Source: CAD feature listing. Evaluate the final solid. Frame: model axes, mm. A direction names the side the tool comes from. Give positions to 0.01 mm unless a question says otherwise; leave off trailing zeros. Write each loop counter-clockwise with the first axis right and the second up, starting at its lowest first coordinate (ties: lowest second). Pieces come first, ordered by that corner, then holes.
Autodesk Inventor part; units mm, degrees
ref_plane "YZ Plane" through (0, 0, 0) normal (1, 0, 0) x (0, 1, 0)
ref_plane "XZ Plane" through (0, 0, 0) normal (0, 1, 0) x (-1, 0, 0)
ref_plane "XY Plane" through (0, 0, 0) normal (0, 0, 1) x (1, 0, 0)
sketch "Sketch1" plane through (0, 0, 0) normal (0, 0, 1) x (1, 0, 0)
  line L0 (-79, -26.3395) -> (-79, 33.1605)
  line L1 (-1.5, -26.3395) -> (-79, -26.3395)
  line L2 (-1.5, -9.5895) -> (-1.5, -26.3395)
  line L3 (-1.5, 8.4105) -> (-1.5, -1.5895)
  line L4 (-1.5, 33.1605) -> (-1.5, 16.4105)
  line L5 (-79, 33.1605) -> (-1.5, 33.1605)
  line L6 (-1.5, -9.5895) -> (-1.5, -1.5895)
  line L7 (-1.5, 8.4105) -> (-1.5, 16.7071)
  line L8 (-74, -21.3395) -> (-60.5, -21.3395) construction
  line L9 (-74, -7.8395) -> (-74, -21.3395) construction
  line L10 (-60.5, -7.8395) -> (-74, -7.8395) construction
  line L11 (-60.5, -21.3395) -> (-60.5, -7.8395) construction
  line L12 (-74, -3.3395) -> (-60.5, -3.3395) construction
  line L13 (-74, 10.1605) -> (-74, -3.3395) construction
  line L14 (-60.5, 10.1605) -> (-74, 10.1605) construction
  line L15 (-60.5, 10.1605) -> (-74, 10.1605) construction
  line L16 (-60.5, -3.3395) -> (-60.5, 10.1605) construction
  line L17 (-74, 14.6605) -> (-60.5, 14.6605) construction
  line L18 (-74, 28.1605) -> (-74, 14.6605) construction
  line L19 (-60.5, 28.1605) -> (-74, 28.1605) construction
  line L20 (-60.5, 14.6605) -> (-60.5, 28.1605) construction
  line L21 (-79, -18.5895) -> (-82, -18.5895)
  line L22 (-82, -18.5895) -> (-82, -10.5895)
  line L23 (-82, -10.5895) -> (-79, -10.5895)
  line L24 (-79, -0.5895) -> (-82, -0.5895)
  line L25 (-82, -0.5895) -> (-82, 7.4105)
  line L26 (-82, 7.4105) -> (-79, 7.4105)
  line L27 (-79, 17.4105) -> (-82, 17.4105)
  line L28 (-82, 17.4105) -> (-82, 25.4105)
  line L29 (-82, 25.4105) -> (-79, 25.4105)
  line L30 (-82, -9.5895) -> (-82, -1.5895) construction
  line L31 (1.5, -1.5895) -> (1.5, -9.5895) construction
  line L32 (-10.3701, -14.5895) -> (-89.08, -14.5895) construction
  line L33 (-89.5983, 3.4105) -> (-12.2572, 3.4105) construction
  line L34 (-89.5983, 21.4105) -> (-12.2572, 21.4105) construction
  line L35 (-1.5, -18.5895) -> (1.5, -18.5895)
  line L36 (1.5, -18.5895) -> (1.5, -10.5895)
  line L37 (1.5, -10.5895) -> (-1.5, -10.5895)
  line L38 (-1.5, -0.5895) -> (1.5, -0.5895)
  line L39 (1.5, -0.5895) -> (1.5, 7.4105)
  line L40 (1.5, 7.4105) -> (-1.5, 7.4105)
  line L41 (-1.5, 17.4105) -> (1.5, 17.4105)
  line L42 (1.5, 17.4105) -> (1.5, 25.4105)
  line L43 (1.5, 25.4105) -> (-1.5, 25.4105)
  point P0 (0, 0)
  point P1 (-74, -14.5895)
  point P2 (-74, 3.4105)
  point P3 (-74, 21.4105)
  point P4 (-82, -14.5895)
  point P5 (-82, 3.4105)
  point P6 (-82, 21.4105)
  point P7 (1.5, -14.5895)
  point P8 (1.5, 3.4105)
  point P9 (1.5, 21.4105)
extrude "Extrusion1" add sketch "Sketch1" against normal blind 3
properties part number "Bottom" material "Polycarbonate, Clear"
1. Pin query (flat end, axial travel): P1, Ø0.9, axis at x = -0.5, z = -1, coming from the +Y side; P2, Ø3, axis at x = -10.5, y = 21.5, coming from the +Z side; P3, Ø1.5, axis at y = -7.5, z = -1, coming from the -X side; P4, Ø1.5, axis at x = 0, z = -1, coming from the -Y side. Return the tip coordinate at first contact, or that it passes through.
2. Access query for faces 1 (the flat face through (-79, -23, -1)), 2 (the flat face through (0, -18.59, -1)), 3 (the flat face through (-80, -0.59, -1)), 4 (the flat face through (0, -10.59, -1)). Directions: +Z, -Z, +X, -X, +Y, -Y. A direction counts if a zero-diameter tool reaches every point of the face in a straight line with its end or side. Return the directions, or none.
3. Section query B-B (y = -6.5). Return loops of the section in (x, z).
4. Section query A-A (z = -1.7). Return loops of the section in (x, y), plus the area to 3 significant figures.
5. Line query: probe 1 along X at (y, z) = (-5.5, -0.6). Output: solid intervals per line, ascending.
The answers:
1. P1: stops at y = 25.41
1. P2: stops at z = 0
1. P3: stops at x = -79
1. P4: stops at y = -18.59
2. face 1: +Z, -Z, -X, -Y
2. face 2: +Z, -Z, +X, -Y
2. face 3: +Z, -Z, -X
2. face 4: +Z, -Z, +X
3. outline: (-79, -3) - (-1.5, -3) - (-1.5, 0) - (-79, 0) - close
4. outline: (-82, -18.59) - (-79, -18.59) - (-79, -26.34) - (-1.5, -26.34) - (-1.5, -18.59) - (1.5, -18.59) - (1.5, -10.59) - (-1.5, -10.59) - (-1.5, -0.59) - (1.5, -0.59) - (1.5, 7.41) - (-1.5, 7.41) - (-1.5, 17.41) - (1.5, 17.41) - (1.5, 25.41) - (-1.5, 25.41) - (-1.5, 33.16) - (-79, 33.16) - (-79, 25.41) - (-82, 25.41) - (-82, 17.41) - (-79, 17.41) - (-79, 7.41) - (-82, 7.41) - (-82, -0.59) - (-79, -0.59) - (-79, -10.59) - (-82, -10.59) - close
4. area: 4,760 mm2
5. probe 1: x = -79 to -1.5
